```python
from build123d import *

# Parameters (mm, degrees)
F1_DEPTH       = 19.05
F3_D           = 15.0114
F3_DEPTH       = 14.224
F3_TIP         = 4.5098795482
F6_D           = 8.001
F6_DEPTH       = 25.4
F6_TIP         = 2.4037429064
F6_ON_F5_D     = 8.001
F6_ON_F5_DEPTH = 25.4
F6_ON_F5_TIP   = 2.4037429064
F8_D           = 8.001
F8_DEPTH       = 14.224
F8_TIP         = 2.4037429064
F10_D          = 8.001
F10_DEPTH      = 41.275
F10_TIP        = 2.4037429064


with BuildPart() as f1:
    # F0 (on Front) → F1 (new body)
    with BuildSketch(Plane.XZ):
        Polygon((-304.8, -342.9), (304.8, -342.9), (304.8, 342.9), (50.8, 342.9), (50.8, 292.1), (-50.8, 292.1), (-50.8, 342.9), (-304.8, 342.9), align=None)
    extrude(amount=F1_DEPTH)

    # F3
    with Locations(Plane.XZ.offset(19.05)):
        with Locations((-228.6, 319.024), (228.6, 319.024)):
            Hole(F3_D / 2, depth=F3_DEPTH)
            with Locations((0, 0, -(F3_DEPTH + F3_TIP / 2))):  # 118° drill point
                Cone(0, F3_D / 2, F3_TIP, mode=Mode.SUBTRACT)

    # F6
    with Locations(Plane.XY.offset(342.9)):
        with Locations((-228.6, -9.525)):
            Hole(F6_D / 2, depth=F6_DEPTH)
            with Locations((0, 0, -(F6_DEPTH + F6_TIP / 2))):  # 118° drill point
                Cone(0, F6_D / 2, F6_TIP, mode=Mode.SUBTRACT)

    # F6 on F5
    with Locations(Plane.XY.offset(342.9)):
        with Locations((228.6, -9.525)):
            Hole(F6_ON_F5_D / 2, depth=F6_ON_F5_DEPTH)
            with Locations((0, 0, -(F6_ON_F5_DEPTH + F6_ON_F5_TIP / 2))):  # 118° drill point
                Cone(0, F6_ON_F5_D / 2, F6_ON_F5_TIP, mode=Mode.SUBTRACT)

    # F8
    with Locations(Plane.XZ.offset(19.05)):
        with Locations((-295.275, 292.1), (-295.275, 0), (-295.275, -292.1), (295.275, -292.1), (295.275, 0), (295.275, 292.1)):
            Hole(F8_D / 2, depth=F8_DEPTH)
            with Locations((0, 0, -(F8_DEPTH + F8_TIP / 2))):  # 118° drill point
                Cone(0, F8_D / 2, F8_TIP, mode=Mode.SUBTRACT)

    # F10
    with Locations(Plane(origin=(0, 0, -342.9), x_dir=(1, 0, 0), z_dir=(0, 0, -1))):
        with Locations((-241.3, 9.525), (241.3, 9.525)):
            Hole(F10_D / 2, depth=F10_DEPTH)
            with Locations((0, 0, -(F10_DEPTH + F10_TIP / 2))):  # 118° drill point
                Cone(0, F10_D / 2, F10_TIP, mode=Mode.SUBTRACT)


solid = f1.part
```
Check sheet for the modelled part. Datum: model origin and axes. Units: mm. A direction names the side the tool comes from. Round coordinates to 2 decimals unless told otherwise and drop trailing zeros. Loops run counter-clockwise (first coordinate to the right, second up) from the corner with the lowest first, then second, coordinate; pieces in that order, holes last. Notation, with made-up numbers: (49, 88) - (80, 88) arc R9 ccw to (80, 98) - close; hole circle Ø4 at (-23.75, -28.75). An arc over 180 degrees is marked (long way). Answer as a JSON object with one key per item and string values. Group by question number.
Q1. Set-up check for faces 1 (the face through (-304.8, -9, 5)), 2 (the face through (-226.973, -11.838, 311.697)), 3 (the face through (1, -9, 292.1)): record each of +Z, -Z, +X, -X, +Y, -Y from which the full face is reachable in a straight line by a thin tool's end or side.
Q2. Sectioned sample at A-A, the plane x = -29.5. Enter the section's corners in (y, z), plus the area to 3 significant figures.
Q3. Gauge pin test, flat ends, axial feed: P1, Ø6.5, axis at x = -295.275, z = -292.1, coming from the -Y side; P2, Ø5.5, axis at x = -16, y = -5.5, coming from the +Z side; P3, Ø5, axis at x = 228.6, y = -9.525, coming from the +Z side. Record the tip position at first contact, or that the pin passes through.
Q4. Mould release check, pull along X, two halves, no side actions. Record for faces 4 (the face through (-228.88, -1.1, 317.75)), 5 (the face through (304.8, -9, -5)), 6 (the face through (-4, -19.05, 5)): released by +X, released by -X, zero draft, split by the parting line, or undercut.
Q5. Scan lines: line 1 along X through (y, z) = (-12, -292.1); line 2 along Y through (x, z) = (-228.6, 333); line 3 along Z through (x, y) = (-47, -4.5). Record each from-to range of solid material in increasing order. Write a range as [from, to].
Solution:
{
 "1": {"face 1": "+Z, -Z, -X, +Y, -Y", "face 2": "-Y", "face 3": "+Z, +Y, -Y"},
 "2": {"outline": "(-19.05, -342.9) - (0, -342.9) - (0, 292.1) - (-19.05, 292.1) - close", "area": "12,100 mm²"},
 "3": {"P1": "stops at y = -4.38", "P2": "stops at z = 292.1", "P3": "stops at z = 311.95"},
 "4": {"face 4": "undercut", "face 5": "released by +X", "face 6": "zero draft"},
 "5": {"line 1": "x = [-304.8, -299.28], [-291.27, 291.27], [299.28, 304.8]", "line 2": "y = [-19.05, -13.53], [-5.52, 0]", "line 3": "z = [-342.9, 292.1]"}
}
